```python
from build123d import *

# Parameters (mm, degrees)
BOSS_EXTRUDE1_DEPTH = 6
SKETCH2_R           = 5
CUT_EXTRUDE1_DEPTH  = 6
SCALE1_SCALE        = 0.3


with BuildPart() as part:
    # Sketch1 → Boss-Extrude1 (new body)
    with BuildSketch(Plane.XY):
        with BuildLine():
            Line((-13.846153846, 7), (16.153846154, 7))
            ThreePointArc((16.153846154, 7), (23.153846154, 0), (16.153846154, -7))
            Line((16.153846154, -7), (-13.846153846, -7))
            ThreePointArc((-13.846153846, -7), (-20.846153846, 0), (-13.846153846, 7))
        make_face()
    extrude(amount=BOSS_EXTRUDE1_DEPTH)

    # Sketch2 → Cut-Extrude1 (cut)
    with BuildSketch(Plane.XY.offset(6)):
        with Locations((-13.846153846, 0)):
            Circle(SKETCH2_R)
        with Locations((16.153846154, 0)):
            Circle(SKETCH2_R)
    extrude(amount=-CUT_EXTRUDE1_DEPTH, mode=Mode.SUBTRACT)


with BuildPart() as part_1:
    # Scale1: scaled about (1.153846154, 0, 3)
    add(part.part.scale(SCALE1_SCALE).moved(Location((0.807692308, 0, 2.1))))


solid = part_1.part
```
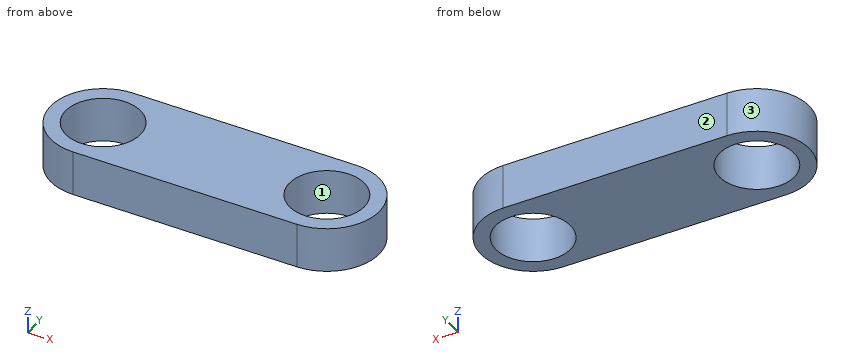
Can you work these out from the model? Positions are in its coordinate system, mm. Face numbers are marked on the shaded views. Coordinates: 2 decimals unless noted, no trailing zeros. Write each loop counter-clockwise with the first axis right and the second up, starting at its lowest first coordinate (ties: lowest second). Pieces come first, ordered by that corner, then holes. Notation, with made-up numbers: M -30,-14.75 L -11,-14.75 A16 cw -11,14.25 Z; hole C 27,54.5 d10. An arc over 180 degrees is marked long. Answer as CSV lines item,"result".
Item 1: Imagine slicing it at D-D on y = 0.65. List the corners of the cut face in (x, z) for me, plus the area to 3 significant figures.
Geometry results:
outline,"M -5.34,2.1 L -4.7,2.1 L -4.7,3.9 L -5.34,3.9 Z; M -1.99,2.1 L 4.3,2.1 L 4.3,3.9 L -1.99,3.9 Z; M 7.01,2.1 L 7.65,2.1 L 7.65,3.9 L 7.01,3.9 Z"
area,"13.7 mm2"
Item 2: Imagine slicing it at C-C on x = 5.5. List the corners of the cut face in (y, z) for me.
Geometry results:
outline,"M -2.1,2.1 L -1.49,2.1 L -1.49,3.9 L -2.1,3.9 Z; M 1.49,2.1 L 2.1,2.1 L 2.1,3.9 L 1.49,3.9 Z"
Item 3: Imagine slicing it at B-B on z = 3.4. List the corners of the cut face in (x, y) for me.
Geometry results:
outline,"M -3.35,-2.1 L 5.65,-2.1 A2.1 ccw 5.65,2.1 L -3.35,2.1 A2.1 ccw Z; hole C -3.35,0 d3; hole C 5.65,0 d3"
Item 4: Please list where these lines run through material, in increasing order: line 1 along X through (y, z) = (-0.05, 3.1); line 2 along X through (y, z) = (-0.3, 2.75); line 3 along Y through (x, z) = (5.75, 2.65).
Geometry results:
line 1,"x = -5.45 to -4.85, -1.85 to 4.15, 7.15 to 7.75"
line 2,"x = -5.42 to -4.82, -1.88 to 4.18, 7.12 to 7.73"
line 3,"y = -2.1 to -1.5, 1.5 to 2.1"
Item 5: I'm going to push a flat-ended pin straight in: P1, Ø1, axis at y = -1, z = 2.5, coming from the +X side. Where does the tip first touch, or does it pass through?
Geometry results:
P1,"stops at x = 7.69"
Item 6: Imagine slicing it at A-A on y = 0. List the corners of the cut face in (x, z) for me, plus the area to 3 significant figures.
Geometry results:
outline,"M -5.45,2.1 L -4.85,2.1 L -4.85,3.9 L -5.45,3.9 Z; M -1.85,2.1 L 4.15,2.1 L 4.15,3.9 L -1.85,3.9 Z; M 7.15,2.1 L 7.75,2.1 L 7.75,3.9 L 7.15,3.9 Z"
area,"13.0 mm2"
Item 7: We'd pull the mould along X, two halves only. Please class the marked faces 1, 2 and 3: +X half, -X half, draft (parallel to the pull), parting line (faces both ways), or undercut.
Geometry results:
face 1,"undercut"
face 2,"draft"
face 3,"-X half"
